Verification items for the finished model (mm, model axes). A direction names the side the tool comes from. Coordinates: 2 decimals unless noted, no trailing zeros. Loops run counter-clockwise (first coordinate to the right, second up) from the corner with the lowest first, then second, coordinate; pieces in that order, holes last. Notation, with made-up numbers: (15, 19) - (20, 19) arc R21 cw to (20, 43) - close; hole circle Ø7 at (-34.5, 75). An arc over 180 degrees is marked (long way). One line per item, written item: value. Start each with the question number.
(1) Section check C-C (x = -98.5). Record the boundary of the cut face in (y, z), plus the area to 3 significant figures.
(2) Section check B-B (z = 42.5). Record the boundary of the cut face in (x, y), plus the area to 3 significant figures.
(3) Section check D-D (x = -41). Record the boundary of the cut face in (y, z), plus the area to 3 significant figures.
(4) Gauge pin test, flat ends, axial feed: P1, Ø4, axis at x = -43.5, y = 89, coming from the -Z side; P2, Ø4, axis at x = -71.5, y = 93, coming from the -Z side; P3, Ø12, axis at x = -49, y = 38, coming from the +Z side; P4, Ø5.5, axis at x = 0, z = 0, coming from the -Y side. Record the tip position at first contact, or that the pin passes through.
(5) Section check A-A (y = 111). Record the boundary of the cut face in (x, z) (3 decimals), plus the area to 3 significant figures.
(6) Set-up check for faces 1 (the face through (-12, 63, 46.685)), 2 (the face through (-86, 63, -3.226)), 3 (the face through (-12, 63, 49.225)), 4 (the face through (-86, 63, -0.686)), 5 (the face through (-41.877, 62.611, 21.97)): record each of +Z, -Z, +X, -X, +Y, -Y from which the full face is reachable in a straight line by a thin tool's end or side.
(7) Thickness scan on probe 1 along Z at (x, y) = (0, 96) (3 decimals); probe 2 along X at (y, z) = (69, 6); probe 3 along X at (y, z) = (9, 16). Record the ranges inside material, lowest first. Write a range as [from, to].
```python
from build123d import *

# Parameters (mm, degrees)
F0_R     = 3.175
F1_DEPTH = 127
F2_R     = 5.08
F3_R     = 2.54


with BuildPart() as f1:
    # F0 (on Front) → F1 (new body)
    with BuildSketch(Plane.XZ):
        with BuildLine():
            ThreePointArc((2.4511, 4.34778), (4.309569, 2.517677), (4.9911, 0))
            Line((4.9911, 0), (4.9911, 49.2252))
            Line((4.9911, 49.2252), (-26.7589, 49.2252))
            Line((-26.7589, 49.2252), (-60.0329, -0.6858))
            Line((-60.0329, -0.6858), (-110.8329, -0.6858))
            Line((-110.8329, -0.6858), (-110.8329, -3.2258))
            Line((-110.8329, -3.2258), (-58.673533, -3.2258))
            Line((-58.673533, -3.2258), (-25.399533, 46.6852))
            Line((-25.399533, 46.6852), (2.4511, 46.6852))
            Line((2.4511, 46.6852), (2.4511, 4.34778))
        make_face()
        with BuildLine():
            ThreePointArc((2.4511, 4.34778), (-4.309569, -2.517677), (4.9911, 0))
            ThreePointArc((4.9911, 0), (4.309569, 2.517677), (2.4511, 4.34778))
        make_face()
        Circle(F0_R, mode=Mode.SUBTRACT)
    extrude(amount=-F1_DEPTH)

    # F2
    f2_edges = [f1.edges().sort_by_distance(p)[0] for p in [
        (-26.7589, 63.5, 49.2252),
        (4.9911, 63.5, 49.2252),
        (-58.673533, 63.5, -3.2258),
    ]]
    fillet(f2_edges, radius=F2_R)

    # F3
    f3_edges = [f1.edges().sort_by_distance(p)[0] for p in [
        (2.4511, 63.5, 46.6852),
        (-25.399533, 63.5, 46.6852),
        (-60.0329, 63.5, -0.6858),
    ]]
    fillet(f3_edges, radius=F3_R)


solid = f1.part
```
Responses:
1. outline: (0, -3.23) - (127, -3.23) - (127, -0.69) - (0, -0.69) - close
1. area: 323 mm²
2. outline: (-31.24, 0) - (-28.19, 0) - (-28.19, 127) - (-31.24, 127) - close; (2.45, 0) - (4.99, 0) - (4.99, 127) - (2.45, 127) - close
2. area: 710 mm²
3. outline: (0, 23.28) - (127, 23.28) - (127, 27.86) - (0, 27.86) - close
3. area: 582 mm²
4. P1: stops at z = 16.53
4. P2: stops at z = -3.23
4. P3: stops at z = 24.86
4. P4: passes through
5. outline: (-110.833, -3.226) - (-61.392, -3.226) arc R5.08 ccw to (-57.165, -0.964) - (-26.154, 45.554) arc R2.54 cw to (-24.04, 46.685) - (-0.089, 46.685) arc R2.54 cw to (2.451, 44.145) - (2.451, 4.348) arc R4.991 ccw (long way) to (4.991, 0) - (4.991, 44.145) arc R5.08 ccw to (-0.089, 49.225) - (-24.04, 49.225) arc R5.08 ccw to (-28.267, 46.963) - (-59.279, 0.445) arc R2.54 cw to (-61.392, -0.686) - (-110.833, -0.686) - close; hole circle Ø6.35 at (0, 0)
5. area: 514 mm²
6. face 1: +Y, -Y
6. face 2: -Z, -X, +Y, -Y
6. face 3: +Z, +X, -X, +Y, -Y
6. face 4: +Z, -X, +Y, -Y
6. face 5: -Z, +Y, -Y
7. probe 1: z = [-4.991, -3.175], [3.175, 4.991], [46.684, 49.224]
7. probe 2: x = [-55.58, -52.52], [2.45, 4.99]
7. probe 3: x = [-48.91, -45.86], [2.45, 4.99]
